from build123d import *

# Parameters (mm, degrees)
SKETCH_1_W          = 13.5
SKETCH_1_H          = 16
EXTRUDE_1_DEPTH     = 6.2
SKETCH_2_R          = 1.5
EXTRUDE_2_DEPTH     = 2.1
SKETCH_3_W          = 1
SKETCH_3_H          = 6.2
EXTRUDE_3_DEPTH     = 3.3
CUT_EXTRUDE_1_DEPTH = 4
SKETCH_6_W          = 1
SKETCH_6_H          = 6.2
EXTRUDE_4_DEPTH     = 3.3
CUT_EXTRUDE_2_DEPTH = 4


with BuildPart() as part:
    # 草图1 → 凸台-拉伸1 (new body)
    with BuildSketch(Plane(origin=(0, 0, 0), x_dir=(1, 0, 0), z_dir=(0, 1, 0))):
        with Locations((-9.627906977, -0.837209302)):
            Rectangle(SKETCH_1_W, SKETCH_1_H)
    extrude(amount=EXTRUDE_1_DEPTH)

    # 草图2 → 凸台-拉伸2 (add)
    with BuildSketch(Plane.XY.offset(8.837209302)):
        with Locations((-13.399361956, 3.148420963)):
            Circle(SKETCH_2_R)
    extrude(amount=EXTRUDE_2_DEPTH)

    # 草图3 → 凸台-拉伸3 (add)
    with BuildSketch(Plane.ZY.offset(16.377906977)):
        with Locations((3.837209302, 3.1)):
            Rectangle(SKETCH_3_W, SKETCH_3_H)
    extrude(amount=EXTRUDE_3_DEPTH)

    # 草图5 → 切除-拉伸1 (cut)
    with BuildSketch(Plane.XY.offset(4.337209302)):
        with BuildLine():
            ThreePointArc((-19.677906977, 3.1), (-19.421721194, 4.728649747), (-18.677906977, 6.2))
            Line((-18.677906977, 6.2), (-19.677906977, 6.2))
            Line((-19.677906977, 6.2), (-19.677906977, 3.1))
        make_face()
        with BuildLine():
            ThreePointArc((-18.677906977, 0), (-19.421721194, 1.471350253), (-19.677906977, 3.1))
            Line((-19.677906977, 3.1), (-19.677906977, 0))
            Line((-19.677906977, 0), (-18.677906977, 0))
        make_face()
    extrude(amount=-CUT_EXTRUDE_1_DEPTH, mode=Mode.SUBTRACT)

    # 草图6 → 凸台-拉伸4 (add)
    with BuildSketch(Plane(origin=(-2.877906977, 0, 0), x_dir=(0, 0, -1), z_dir=(1, 0, 0))):
        with Locations((-3.837209302, 3.1)):
            Rectangle(SKETCH_6_W, SKETCH_6_H)
    extrude(amount=EXTRUDE_4_DEPTH)

    # 草图10 → 切除-拉伸2 (cut)
    with BuildSketch(Plane.XY.offset(4.337209302)):
        with BuildLine():
            Line((0.422093023, 0), (0.422093023, 2.47192447))
            ThreePointArc((0.422093023, 2.47192447), (0.315811593, 1.218073092), (0, 0))
            Line((0, 0), (0.422093023, 0))
        make_face()
        with BuildLine():
            Line((0.422093023, 6.2), (-0.577906977, 6.2))
            ThreePointArc((-0.577906977, 6.2), (0.167750994, 4.401856278), (0.422093023, 2.47192447))
            Line((0.422093023, 2.47192447), (0.422093023, 6.2))
        make_face()
    extrude(amount=-CUT_EXTRUDE_2_DEPTH, mode=Mode.SUBTRACT)


solid = part.part
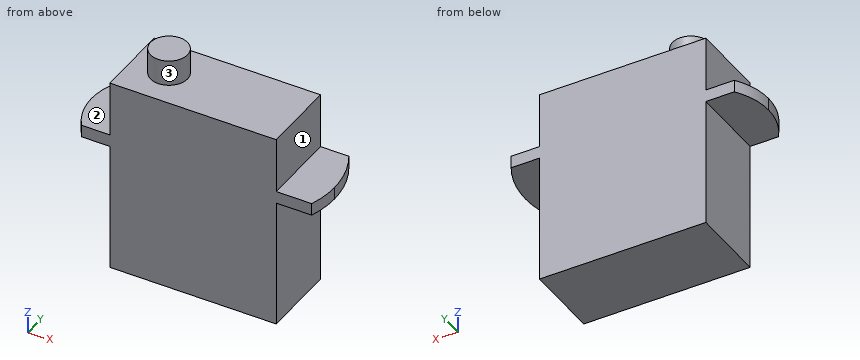
Check sheet for the modelled part. Datum: model origin and axes. Units: mm. Face numbers are marked on the shaded views. A direction names the side the tool comes from. Give positions to 0.01 mm unless a question says otherwise; leave off trailing zeros. Write each loop counter-clockwise with the first axis right and the second up, starting at its lowest first coordinate (ties: lowest second). Pieces come first, ordered by that corner, then holes. Notation, with made-up numbers: (-35.75, 14) -> (-11.75, 14) arc R8 ccw to (-11.75, 26) -> close; hole circle Ø1 at (-34, 9.5). An arc over 180 degrees is marked (long way). Write item = value, one per line.
Item 1: Sectioned sample at B-B on y = 4.25. Record the boundary of the cut face in (x, z), and give its area (3 significant figures).
Output:
outline = (-19.55, 3.34) -> (-16.38, 3.34) -> (-16.38, -7.16) -> (-2.88, -7.16) -> (-2.88, 3.34) -> (0.21, 3.34) -> (0.21, 4.34) -> (-2.88, 4.34) -> (-2.88, 8.84) -> (-12.38, 8.84) -> (-12.38, 10.94) -> (-14.42, 10.94) -> (-14.42, 8.84) -> (-16.38, 8.84) -> (-16.38, 4.34) -> (-19.55, 4.34) -> close
area = 227 mm^2
Item 2: Scan lines: probe 1 along Z at (x, y) = (-18.25, 5.75); probe 2 along X at (y, z) = (5.5, 6.75); probe 3 along Z at (x, y) = (-4.5, 4). Record each from-to range of solid material in increasing order. Write a range as from..to.
Output:
probe_1 = 3.34..4.34
probe_2 = -16.38..-2.88
probe_3 = -7.16..8.84
Item 3: Gauge pin test, flat ends, axial feed: pin 1 (3.5 mm diameter, centred on x = -17.5, y = 3.5, fed in from +Z); pin 2 (1.7 mm diameter, centred on x = -18, y = 3.5, fed in from -Z); pin 3 (2 mm diameter, centred on y = 3, z = -5.5, fed in from +X). Record the tip position at first contact, or that the pin passes through.
Output:
pin_1 = 8.84
pin_2 = 3.34
pin_3 = -2.88
Item 4: Sectioned sample at A-A on x = -10.5. Record the boundary of the cut face in (y, z), and give its area (3 significant figures).
Output:
outline = (0, -7.16) -> (6.2, -7.16) -> (6.2, 8.84) -> (0, 8.84) -> close
area = 99.2 mm^2
Item 5: Sectioned sample at D-D on y = 1. Record the boundary of the cut face in (x, z), and give its area (3 significant figures).
Output:
outline = (-19.24, 3.34) -> (-16.38, 3.34) -> (-16.38, -7.16) -> (-2.88, -7.16) -> (-2.88, 3.34) -> (0.28, 3.34) -> (0.28, 4.34) -> (-2.88, 4.34) -> (-2.88, 8.84) -> (-16.38, 8.84) -> (-16.38, 4.34) -> (-19.24, 4.34) -> close
area = 222 mm^2
Item 6: Sectioned sample at C-C on z = -1.25. Record the boundary of the cut face in (x, y), and give its area (3 significant figures).
Output:
outline = (-16.38, 0) -> (-2.88, 0) -> (-2.88, 6.2) -> (-16.38, 6.2) -> close
area = 83.7 mm^2
Item 7: Tool access check on the marked faces 1, 2 and 3. Record the directions out of +Z, -Z, +X, -X, +Y, -Y that give a thin tool (end or side, any length) a straight path to the whole face; none if there is none.
Output:
face_1 = +Z, +X, +Y, -Y
face_2 = +Z, -X, +Y, -Y
face_3 = +Z
